Can you work these out from the drawing? Everything is in mm from the part's minimum corner. Coordinates: 2 decimals unless noted, no trailing zeros. Order: outer loops, then holes, each group sorted by start corner. A loop starts at its lowest first (then second) coordinate and runs counter-clockwise, first axis right, second up. Notation, with made-up numbers: (31.25, -3) - (82.25, -3) arc R21 ccw to (82.25, 20) - close; hole circle Ø7 at (-24, 58). An arc over 180 degrees is marked (long way). One line per item, written item: value.
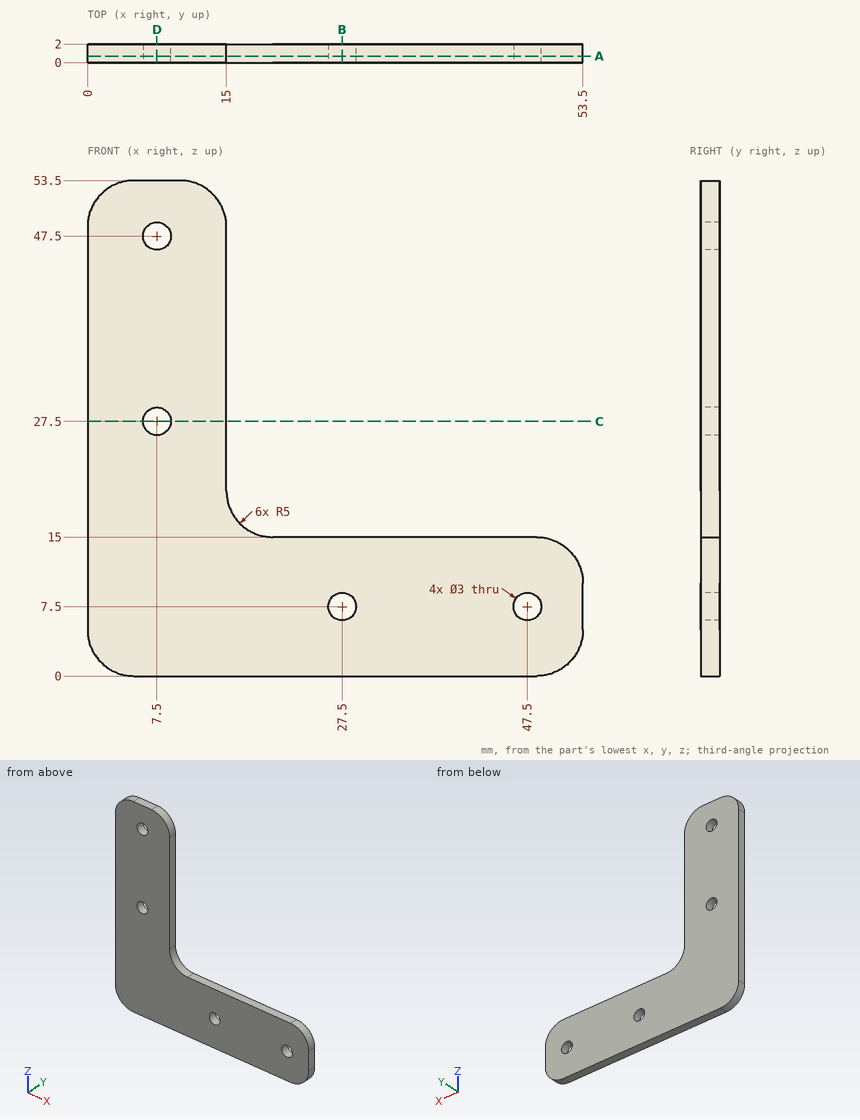
Item 1: I want a section at A-A on y = 0.7. Please give me the cut outline in (x, z).
Conclusion:
outline: (0, 5) arc R5 ccw to (5, 0) - (48.5, 0) arc R5 ccw to (53.5, 5) - (53.5, 10) arc R5 ccw to (48.5, 15) - (20, 15) arc R5 cw to (15, 20) - (15, 48.5) arc R5 ccw to (10, 53.5) - (5, 53.5) arc R5 ccw to (0, 48.5) - close; hole circle Ø3 at (7.5, 27.5); hole circle Ø3 at (7.5, 47.5); hole circle Ø3 at (27.5, 7.5); hole circle Ø3 at (47.5, 7.5)
Item 2: I want a section at B-B on x = 27.5. Please give me the cut outline in (y, z).
Conclusion:
outline: (0, 0) - (2, 0) - (2, 6) - (0, 6) - close; (0, 9) - (2, 9) - (2, 15) - (0, 15) - close
Item 3: I'm going to push flat-ended pins straight in: pin 1 Ø2.5 at (x, z) = (47.5, 7.5) entering from +Y; pin 2 Ø1 at (y, z) = (1, 32.5) entering from +X. Where does each tip first touch, or does it pass through?
Conclusion:
pin 1: through
pin 2: x = 15
Item 4: I want a section at C-C on z = 27.5. Please give me the cut outline in (x, y).
Conclusion:
outline: (0, 0) - (6, 0) - (6, 2) - (0, 2) - close; (9, 0) - (15, 0) - (15, 2) - (9, 2) - close
Item 5: I want a section at D-D on x = 7.5. Please give me the cut outline in (y, z), then the cut area to 3 significant figures.
Conclusion:
outline: (0, 0) - (2, 0) - (2, 26) - (0, 26) - close; (0, 29) - (2, 29) - (2, 46) - (0, 46) - close; (0, 49) - (2, 49) - (2, 53.5) - (0, 53.5) - close
area: 95.0 mm²
Item 6: If I drill on probe 1 along Z at (x, y) = (7.5, 0.75); probe 2 along Z at (x, y) = (47.5, 1), over which ranges is the centre line in solid material (lowest first)?
Conclusion:
probe 1: 0 to 26, 29 to 46, 49 to 53.5
probe 2: 0 to 6, 9 to 15
